Check sheet for the drawn part. Datum: minimum x, y, z corner. Units: mm. Round coordinates to 2 decimals unless told otherwise and drop trailing zeros. Write each loop counter-clockwise with the first axis right and the second up, starting at its lowest first coordinate (ties: lowest second). Pieces come first, ordered by that corner, then holes. Notation, with made-up numbers: M -36,18 L 1,18 A22 ccw 1,41 Z; hole C 69.5,53 d3. An arc over 180 degrees is marked long. Answer in a Markdown table with one row per item. Add a question column.
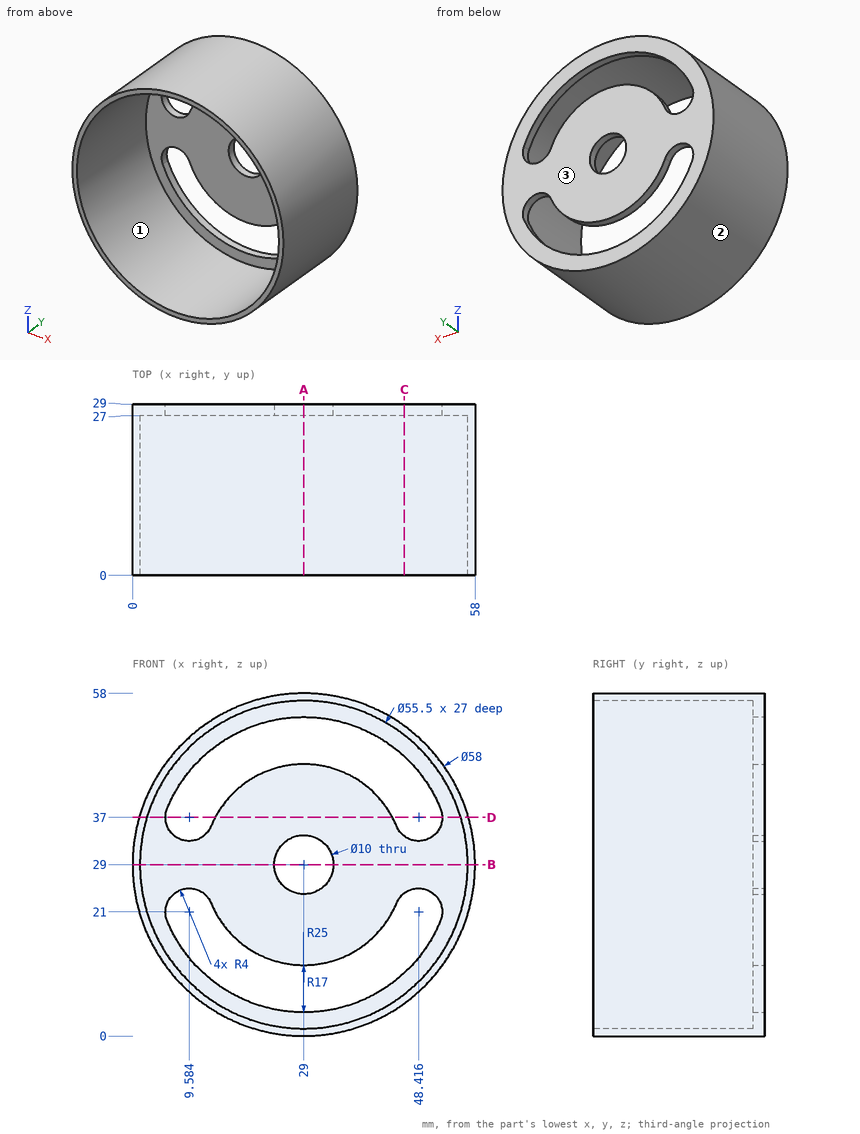
Item 1: Section check A-A, the plane x = 29. Record the boundary of the cut face in (y, z).
Item 2: Section check B-B, the plane z = 29. Record the boundary of the cut face in (x, y).
Item 3: Mould release check, pull along X, two halves, no side actions. Record for the marked faces 1, 2 and 3: +X half, -X half, draft (parallel to the pull), parting line (faces both ways), or undercut.
Item 4: Scan lines: probe 1 along Z at (x, y) = (29, 27.7); probe 2 along Y at (x, z) = (38, 15); probe 3 along Z at (x, y) = (41.5, 25.25) (1 decimal). Record each from-to range of solid material in increasing order. Write a range as from..to.
Item 5: Section check D-D, the plane z = 37. Record the boundary of the cut face in (x, y) (1 decimal), and give its area (3 significant figures).
Item 6: Gauge pin test, flat ends, axial feed: pin 1 Ø6 at (y, z) = (16, 10.5) entering from +X; pin 2 Ø6 at (x, y) = (32.5, 7) entering from +Z; pin 3 Ø5 at (y, z) = (6.5, 16.5) entering from -X; pin 4 Ø8 at (x, z) = (29, 29) entering from -Y. Record the tip position at first contact, or that the pin passes through.
Item 7: Section check C-C, the plane x = 46. Record the boundary of the cut face in (y, z) (1 decimal).
Result sheet:
| question | item | result |
|---|---|---|
| 1 | outline | M 0,0 L 29,0 L 29,4 L 27,4 L 27,1.25 L 0,1.25 Z; M 0,56.75 L 27,56.75 L 27,54 L 29,54 L 29,58 L 0,58 Z; M 27,12 L 29,12 L 29,24 L 27,24 Z; M 27,34 L 29,34 L 29,46 L 27,46 Z |
| 2 | outline | M 0,0 L 1.25,0 L 1.25,27 L 24,27 L 24,29 L 0,29 Z; M 34,27 L 56.75,27 L 56.75,0 L 58,0 L 58,29 L 34,29 Z |
| 3 | face 1 | undercut |
| 3 | face 2 | parting line |
| 3 | face 3 | draft |
| 4 | probe 1 | z = 0..4, 12..24, 34..46, 54..58 |
| 4 | probe 2 | y = 27..29 |
| 4 | probe 3 | z = 2.8..4.2, 53.8..55.2 |
| 5 | outline | M 1.1,0 L 2.4,0 L 2.4,27 L 5.6,27 L 5.6,29 L 1.1,29 Z; M 14,27 L 44,27 L 44,29 L 14,29 Z; M 52.4,27 L 55.6,27 L 55.6,0 L 56.9,0 L 56.9,29 L 52.4,29 Z |
| 5 | area | 148 mm^2 |
| 6 | pin 1 | stops at x = 53.51 |
| 6 | pin 2 | stops at z = 58 |
| 6 | pin 3 | stops at x = 1.78 |
| 6 | pin 4 | passes through |
| 7 | outline | M 0,5.5 L 29,5.5 L 29,10.7 L 27,10.7 L 27,7.1 L 0,7.1 Z; M 0,50.9 L 27,50.9 L 27,47.3 L 29,47.3 L 29,52.5 L 0,52.5 Z; M 27,24.2 L 29,24.2 L 29,33.8 L 27,33.8 Z |
